The model under review builds one solid part; all positions refer to its coordinate system, in mm. Coordinates: 2 decimals unless noted, no trailing zeros. Loops run counter-clockwise (first coordinate to the right, second up) from the corner with the lowest first, then second, coordinate; pieces in that order, holes last. Notation, with made-up numbers: M 79.5,-12 L 99.5,-12 A17 ccw 99.5,4 Z; hole C 25.5,37 d5. An arc over 180 degrees is marked long. Return JSON: item names as keys, results as strings.
```python
from build123d import *

# Parameters (mm, degrees)
BOSS_EXTRUDE1_DEPTH = 74.5
SKETCH2_R           = 4.125
CUT_EXTRUDE1_DEPTH  = 78.783352975


with BuildPart() as part:
    # Sketch1 → Boss-Extrude1 (new, symmetric)
    with BuildSketch(Plane.XY):
        Polygon((-20, 10), (10, 10), (20, 0), (-20, 0), align=None)
    extrude(amount=BOSS_EXTRUDE1_DEPTH, both=True)

    # Sketch2 → Cut-Extrude1 (cut, through all)
    with BuildSketch(Plane(origin=(0, 10, 0), x_dir=(1, 0, 0), z_dir=(0, 1, 0))):
        with Locations(Location((-5.375, 0, 0), (0, 0, 180))):
            Circle(SKETCH2_R)
        with Locations(Location((-5.375, -55, 0), (0, 0, 180))):
            Circle(SKETCH2_R)
        with Locations((-5.375, 55)):
            Circle(SKETCH2_R)
    extrude(amount=-CUT_EXTRUDE1_DEPTH, mode=Mode.SUBTRACT)


solid = part.part
```
1. Add section B-B on y = 6.25. Give the boundary of the cut face in (x, z) (3 decimals), plus the area to 3 significant figures.
Check values:
{"outline": "M -20,-74.5 L 13.75,-74.5 L 13.75,74.5 L -20,74.5 Z; hole C -5.375,-55 d8.25; hole C -5.375,0 d8.25; hole C -5.375,55 d8.25", "area": "4,870 mm²"}
2. Add section D-D on x = 16. Give the boundary of the cut face in (y, z).
Check values:
{"outline": "M 0,-74.5 L 4,-74.5 L 4,74.5 L 0,74.5 Z"}
3. Add section A-A on z = -55. Give the boundary of the cut face in (x, y), plus the area to 4 significant figures.
Check values:
{"outline": "M -20,0 L -9.5,0 L -9.5,10 L -20,10 Z; M -1.25,0 L 20,0 L 10,10 L -1.25,10 Z", "area": "267.5 mm²"}
4. To check wall thickness, follow line 1 (Z direction, x = -5, y = 6.5); line 2 (Z direction, x = -3.5, y = 7.5); line 3 (X direction, y = 4, z = 2). State the ranges of each line that lie inside material, in increasing order.
Check values:
{"line 1": "-74.5 to -59.11, -50.89 to -4.11, 4.11 to 50.89, 59.11 to 74.5", "line 2": "-74.5 to -58.67, -51.33 to -3.67, 3.67 to 51.33, 58.67 to 74.5", "line 3": "-20 to -8.98, -1.77 to 16"}
5. The part is to be moulded in two halves that separate along Z. For faces 1 (the face through (-4, 5, -74.5)), 2 (the face through (-4.481, 5.07, 50.973)), 3 (the face through (15, 5, 1)), say which applies: released by +Z, released by -Z, zero draft, split by the parting line, or undercut.
Check values:
{"face 1": "released by -Z", "face 2": "undercut", "face 3": "zero draft"}
6. Add section C-C on x = -6. Give the boundary of the cut face in (y, z), plus the area to 3 significant figures.
Check values:
{"outline": "M 0,-74.5 L 10,-74.5 L 10,-59.08 L 0,-59.08 Z; M 0,-50.92 L 10,-50.92 L 10,-4.08 L 0,-4.08 Z; M 0,4.08 L 10,4.08 L 10,50.92 L 0,50.92 Z; M 0,59.08 L 10,59.08 L 10,74.5 L 0,74.5 Z", "area": "1,250 mm²"}
